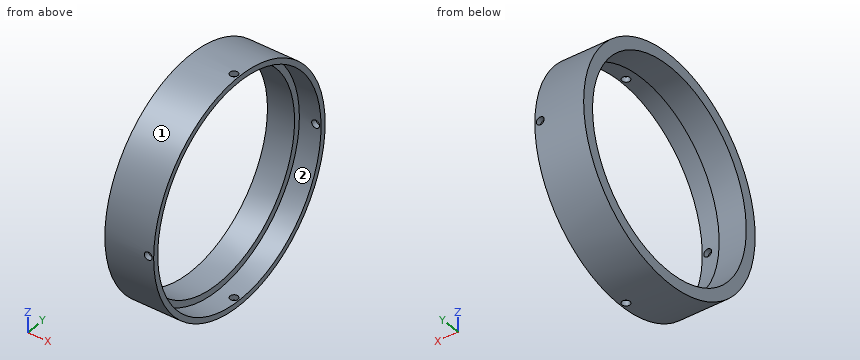
```python
from build123d import *

# Parameters (mm, degrees)
D_GAGEMENT_M2_51_D           = 2.9
R_P_TITION_CIRCULAIRE1_COUNT = 2
R_P_TITION_CIRCULAIRE1_ANGLE = 90


with BuildPart() as part:
    # Esquisse1 → Révolution1 (revolve)
    with BuildSketch(Plane.XY):
        Polygon((0, 42), (0, 37.65), (10, 37.65), (10, 40), (18, 40), (18, 42), align=None)
    revolve(axis=Axis((-19.427138361, 0, 0), (1, 0, 0)))

    # Dégagement M2.51 (through all)
    with Locations(Plane(origin=(16, 42, 0), x_dir=(0, 0, 1), z_dir=(0, 1, 0))):
        with Locations((0, 0)):
            d_gagement_m2_51 = Hole(D_GAGEMENT_M2_51_D / 2)

    # Répétition circulaire1: Dégagement M2.51 ×2 about axis
    r_p_tition_circulaire1_axis = Axis((0, 0, 0), (-1, 0, 0))
    for i in range(1, R_P_TITION_CIRCULAIRE1_COUNT):
        add(d_gagement_m2_51.rotate(r_p_tition_circulaire1_axis, i * R_P_TITION_CIRCULAIRE1_ANGLE / (R_P_TITION_CIRCULAIRE1_COUNT - 1)), mode=Mode.SUBTRACT)


solid = part.part
```
Read the model definition and answer for the solid it produces. Units are mm, in the model's axes. Face numbers are marked on the shaded views. Give positions to 0.01 mm unless a question says otherwise; leave off trailing zeros. Loops run counter-clockwise (first coordinate to the right, second up) from the corner with the lowest first, then second, coordinate; pieces in that order, holes last.
Item 1: Find the intervals of material crossed by line 1 along X through (y, z) = (0, -40.85); line 2 along Z through (x, y) = (3.25, 0); line 3 along Y through (x, z) = (12, -1.5), in increasing order.
Item 2: The mould has two halves that part along Z. Classify the marked faces 1 and 2: released by +Z, released by -Z, zero draft, split by the parting line, or undercut.
Item 3: Each of these flat-tipped pins is pushed along its axis until it touches: pin 1 Ø8 at (x, y) = (14, 9) entering from +Z; pin 2 Ø10 at (x, y) = (14, -9.5) entering from +Z; pin 3 Ø4 at (x, z) = (13.5, -7) entering from +Y; pin 4 Ø12 at (y, z) = (5, 31) entering from +X. Where does it stop, or does it pass through?
Item 4: The part is cut by section C-C (y = -36). Write down the section's boundary in (x, z), and give its area (3 significant figures).
Item 5: The part is cut by section D-D (z = -12.5). Write down the section's boundary in (x, y).
Item 6: The part is cut by section A-A (z = 0). Write down the section's boundary in (x, y), and give its area (3 significant figures).
Taken from the geometry:
1. line 1: x = 0 to 14.55, 17.45 to 18
1. line 2: z = -42 to -37.65, 37.65 to 42
1. line 3: y = -41.97 to -39.97, 39.97 to 41.97
2. face 1: split by the parting line
2. face 2: undercut
3. pin 1: stops at z = 41.7
3. pin 2: stops at z = 41.76
3. pin 3: stops at y = 41.7
3. pin 4: passes through
4. outline: (0, -21.63) - (18, -21.63) - (18, -17.44) - (10, -17.44) - (10, -11.02) - (0, -11.02) - close; (0, 11.02) - (10, 11.02) - (10, 17.44) - (18, 17.44) - (18, 21.63) - (0, 21.63) - close
4. area: 279 mm2
5. outline: (0, -40.1) - (18, -40.1) - (18, -38) - (10, -38) - (10, -35.51) - (0, -35.51) - close; (0, 35.51) - (10, 35.51) - (10, 38) - (18, 38) - (18, 40.1) - (0, 40.1) - close
6. outline: (0, -42) - (14.55, -42) - (14.55, -40) - (10, -40) - (10, -37.65) - (0, -37.65) - close; (0, 37.65) - (10, 37.65) - (10, 40) - (14.55, 40) - (14.55, 42) - (0, 42) - close; (17.45, -42) - (18, -42) - (18, -40) - (17.45, -40) - close; (17.45, 40) - (18, 40) - (18, 42) - (17.45, 42) - close
6. area: 107 mm2
